Geometry: final body of the model. Coordinates: model frame, mm. Face numbers are marked on the shaded views. Round coordinates to 2 decimals unless told otherwise and drop trailing zeros. Loops run counter-clockwise (first coordinate to the right, second up) from the corner with the lowest first, then second, coordinate; pieces in that order, holes last. Notation, with made-up numbers: M -27.75,-2 L -15.75,-2 A17 ccw -15.75,8 Z; hole C -23,-12.75 d2. An arc over 180 degrees is marked long. Answer as a JSON object with one key per item and string values.
Autodesk Inventor part; units mm, degrees
ref_plane "YZ Plane" through (0, 0, 0) normal (1, 0, 0) x (0, 1, 0)
ref_plane "XZ Plane" through (0, 0, 0) normal (0, 1, 0) x (-1, 0, 0)
ref_plane "XY Plane" through (0, 0, 0) normal (0, 0, 1) x (1, 0, 0)
sketch "Sketch1" plane through (0, 0, 0) normal (0, 1, 0) x (-1, 0, 0)
  line L0 (15, 118.75) -> (-15, 118.75)
  line L1 (-15, -118.75) -> (15, -118.75)
  line L2 (15, -118.75) -> (15, 118.75)
  line L3 (15, 118.75) -> (-15, -118.75) construction
  line L4 (-15, 118.75) -> (15, -118.75) construction
  line L5 (-15, 15) -> (-145.33, 15)
  line L6 (15, 0) -> (-145.33, 0) construction
  line L7 (-15, -15) -> (-145.33, -15)
  line L8 (-145.33, 15) -> (-145.33, -15)
  line L9 (-15, 118.75) -> (-15, 15)
  line L10 (-15, -15) -> (-15, -118.75)
  point P0 (0, 0)
  dimension "d0" = 30
  dimension "d1" = 237.5
  dimension "d2" = 15
  dimension "d3" = 130.33
extrude "Extrusion1" add sketch "Sketch1" along normal blind 30
ref_plane "Work Plane1" through (15, 0, 0) normal (0, 0, 1) x (1, 0, 0)
sketch "Sketch2" plane through (0, 30, 0) normal (0, 1, 0) x (1, 0, 0)
  line L0 (-15, 118.75) -> (-15, -118.75)
  line L1 (15, -118.75) -> (15, -15)
  line L2 (-15, -118.75) -> (15, -118.75)
  line L3 (15, -118.75) -> (15, -98.75)
  line L4 (15, -98.75) -> (-15, -98.75)
  line L5 (-15, -98.75) -> (-15, -118.75)
  point P0 (0, 0)
  point P1 (15, -118.75)
  point P2 (-15, -98.75)
  dimension "d6" = 20
extrude "Extrusion2" add sketch "Sketch2" along normal blind 20
sketch "Sketch3" plane through (-15, 0, 118.75) normal (0, 0, 1) x (1, 0, 0)
  line L0 (0, 50) -> (30, 50)
  line L1 (30, 0) -> (30, 50)
  point P0 (15, 0)
  point P1 (15, 42)
  dimension "d9" = 8
  dimension "d10" = 15
hole "Hole1" at (0, 42, 118.75) direction (0, 0, -1) diameter 6 depth 10 tip angle 118 counterbore diameter 9 counterbore depth 5
mirror "Mirror1" about plane through (15, 0, 0) normal (0, 0, 1) of "Extrusion2", "Hole1"
sketch "Sketch4" plane through (145.33, 0, 15) normal (1, 0, 0) x (0, 0, -1)
  line L0 (0, 0) -> (30, 0)
  line L1 (30, 0) -> (30, 30)
  line L2 (0, 30) -> (30, 30)
  line L3 (0, 0) -> (0, 30)
  line L4 (4, 26) -> (26, 26)
  line L5 (26, 26) -> (26, 4)
  line L6 (26, 4) -> (4, 4)
  line L7 (4, 4) -> (4, 26)
  point P0 (15, 0)
extrude "Extrusion3" cut sketch "Sketch4" against normal blind 65 contours L4 L5 L6 L7
sketch "Sketch5" plane through (15, 0, 15) normal (0, 0, 1) x (1, 0, 0)
  line L0 (65.33, 4) -> (65.33, 26)
  circle A0 centre (82.83, 15) radius 4
  circle A1 centre (112.83, 15) radius 4
  point P0 (-15, 0)
  point P1 (65.33, 15)
  dimension "d20" = 8
  dimension "d21" = 8
  dimension "d22" = 30
  dimension "d23" = 17.5
extrude "Extrusion4" cut sketch "Sketch5" against normal through all
fillet "Fillet1" radius 5 28 edges at (15, 15, 15) (15, 15, -15) (80.165, 0, 15) (80.165, 0, -15) (80.165, 30, -15) (80.165, 30, 15) (15, 30, 56.875) (15, 30, -56.875) (15, 0, -66.875) (15, 0, 66.875) (15, 25, 118.75) (-15, 25, 118.75) (0, 0, 118.75) (-15, 0, 0) (0, 0, -118.75) (15, 25, -118.75) (-15, 25, -118.75) (-15, 30, 0) (15, 50, 108.75) (-15, 50, 108.75) (0, 50, 98.75) (-15, 40, 98.75) (15, 40, 98.75) (15, 40, -98.75) (0, 50, -98.75) (15, 50, -108.75) (-15, 50, -108.75) (-15, 40, -98.75)
sketch "Sketch6" plane through (0, 30, 0) normal (0, 1, 0) x (1, 0, 0)
  line L0 (-10, -98.75) -> (-10, 98.75)
  line L1 (-10, -98.75) -> (10, -98.75)
  point P0 (0, 0)
  point P1 (0, -83.75)
  dimension "d27" = 10
  dimension "d35" = 15
hole "Hole2" at (0, 30, 83.75) direction (0, -1, 0) diameter 6 depth 10 tip angle 118 counterbore diameter 9 counterbore depth 5
sketch "Sketch7" plane through (0, 30, 0) normal (0, 1, 0) x (1, 0, 0)
  line L0 (20, 10) -> (145.33, 10)
  line L1 (-10, -98.75) -> (-10, 98.75)
  line L2 (10, 98.75) -> (-10, 98.75)
  point P0 (0, 0)
  point P1 (0, 83.75)
  point P2 (50, 0)
  dimension "d36" = 10
  dimension "d44" = 60
  dimension "d45" = 10
  dimension "d46" = 15
hole "Hole3" at (50, 30, 0) at (0, 30, -83.75) direction (0, -1, 0) diameter 6 depth 10 tip angle 118 counterbore diameter 9 counterbore depth 5
properties part number "e" material "PCTG 20%"
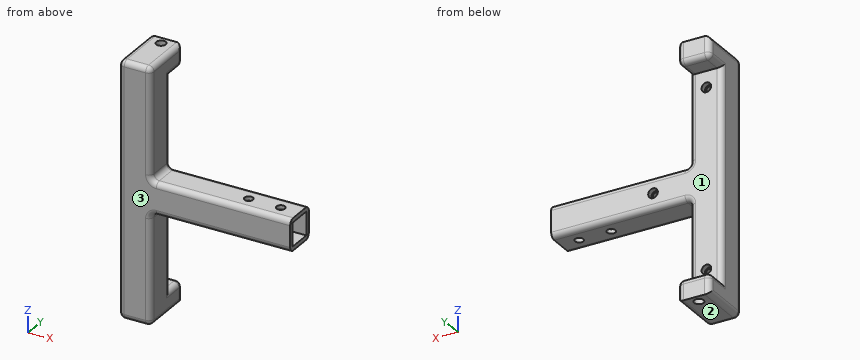
1) Line query: probe 1 along Z at (x, y) = (0, 23); probe 2 along Z at (x, y) = (82, 15); probe 3 along X at (y, z) = (22.8, 0). Output: solid intervals per line, ascending.
Geometry results:
{"probe 1": "-118.75 to -86.75, -80.75 to 80.75, 86.75 to 118.75", "probe 2": "-15 to -11, 11 to 15", "probe 3": "-15 to 47, 53 to 80.33"}
2) Cut plane C-C on z = -91.5. Return the cut outline in (x, y), and give its area (3 significant figures).
Geometry results:
{"outline": "M -15,5 A5 ccw -10,0 L 10,0 A5 ccw 15,5 L 15,25 A5 ccw 10,30 L -10,30 A5 ccw -15,25 Z", "area": "879 mm2"}
3) First-contact query: pin 1 (3 mm diameter, centred on x = 4, z = -50, fed in from +Y); pin 2 (5 mm diameter, centred on x = 21, y = 29.5, fed in from -Z); pin 3 (10.5 mm diameter, centred on x = 97.83, y = 15, fed in from +Z); pin 4 (4 mm diameter, centred on y = 22.5, z = -9.5, fed in from +X). Flat tips, straight axial feed; report the tip coordinate or a pass-through.
Geometry results:
{"pin 1": "y = 30", "pin 2": "z = -14.58", "pin 3": "z = 15", "pin 4": "x = 145.33"}
4) Cut plane B-B on x = 97.83. Return the cut outline in (y, z).
Geometry results:
{"outline": "M 0,-10 A5 ccw 5,-15 L 11,-15 L 11,-11 L 4,-11 L 4,11 L 11,11 L 11,15 L 5,15 A5 ccw 0,10 Z; M 19,-15 L 25,-15 A5 ccw 30,-10 L 30,10 A5 ccw 25,15 L 19,15 L 19,11 L 26,11 L 26,-11 L 19,-11 Z"}
5) Cut plane D-D on x = 32. Return the cut outline in (y, z), and give its area (3 significant figures).
Geometry results:
{"outline": "M 0,-10 A5 ccw 5,-15 L 25,-15 A5 ccw 30,-10 L 30,10 A5 ccw 25,15 L 5,15 A5 ccw 0,10 Z", "area": "879 mm2"}
6) Cut plane A-A on y = 32.5. Return the cut outline in (x, z).
Geometry results:
{"outline": "M -15,-113.75 A5 ccw -10,-118.75 L 10,-118.75 A5 ccw 15,-113.75 L 15,-103.75 A5 ccw 10,-98.75 L -10,-98.75 A5 ccw -15,-103.75 Z; M -15,103.75 A5 ccw -10,98.75 L 10,98.75 A5 ccw 15,103.75 L 15,113.75 A5 ccw 10,118.75 L -10,118.75 A5 ccw -15,113.75 Z"}
7) Pull-direction query (Z, two-part tool) for the marked faces 1, 2 and 3; classes: +Z half, -Z half, draft (parallel to the pull), parting line (faces both ways), or undercut.
Geometry results:
{"face 1": "undercut", "face 2": "-Z half", "face 3": "draft"}
